from build123d import *

# Parameters (mm, degrees)
F0_R     = 5
F1_DEPTH = 3
F2_R     = 15
F3_DEPTH = 3
F4_R     = 17.221585
F5_DEPTH = 25


with BuildPart() as f1:
    # F0 (on Front) → F1 (new body)
    with BuildSketch(Plane.XZ):
        Circle(F0_R)
    extrude(amount=F1_DEPTH)

    # F2 (on face) → F3 (join)
    with BuildSketch(Plane.XZ.offset(3)):
        Circle(F2_R)
    extrude(amount=F3_DEPTH)

    # F4 (on face) → F5 (cut)
    with BuildSketch(Plane.XZ.offset(6)):
        Circle(F4_R)
        Polygon((-9.586422, 12.19146), (-0.589618, 15.497856), (8.6324, 12.884598), (14.557135, 5.349861), (14.921539, -4.228341), (9.586422, -12.19146), (0.589618, -15.497856), (-8.6324, -12.884598), (-14.557135, -5.349861), (-14.921539, 4.228341), align=None, mode=Mode.SUBTRACT)
    extrude(amount=-F5_DEPTH, mode=Mode.SUBTRACT)


solid = f1.part
Here's how the part is built. I have some questions about the finished solid (model axes, mm). Give positions to 0.01 mm unless a question says otherwise; leave off trailing zeros. Loops run counter-clockwise (first coordinate to the right, second up) from the corner with the lowest first, then second, coordinate; pieces in that order, holes last. Notation, with made-up numbers: (78.5, 4.25) -> (112.5, 4.25) arc R8 ccw to (112.5, 14.25) -> close; hole circle Ø9 at (83, -29.75). An arc over 180 degrees is marked (long way). Answer as a JSON object with one key per item and string values. Group by question number.
Item 1: I need wall thicknesses on L1, parallel to Y at x = 6.25, z = 3.75; L2, parallel to X at y = -4.85, z = 2.25; L3, parallel to X at y = -5.8, z = -12.5. Which ranges of each line are inside material? Lowest first, please.
Item 2: Will these pins go through, and if not, where does the flat tip stop? pin 1 (5 mm diameter, centred on x = -3.5, z = -11, fed in from +Y); pin 2 (3 mm diameter, centred on x = 6, y = -2.5, fed in from +Z).
Item 3: Imagine slicing it at B-B on x = 0. Write out the boundary of the cut face in (y, z).
Item 4: Imagine slicing it at C-C on z = 0. Write out the boundary of the cut face in (x, y), then the cut area to 3 significant figures.
Item 5: Imagine slicing it at A-A on y = -3.6. Write out the boundary of the cut face in (x, z).
Item 6: Imagine slicing it at D-D on y = -1.2. Write out the boundary of the cut face in (x, z), then the cut area to 3 significant figures.
Answer list:
{
 "1": {"L1": "y = -6 to -3", "L2": "x = -14.83 to 14.68", "L3": "x = -8.29 to 8.29"},
 "2": {"pin 1": "stops at y = -3", "pin 2": "stops at z = 14.03"},
 "3": {"outline": "(-6, -15) -> (-3, -15) -> (-3, -5) -> (0, -5) -> (0, 5) -> (-3, 5) -> (-3, 15) -> (-6, 15) -> close"},
 "4": {"outline": "(-14.76, -6) -> (14.76, -6) -> (14.76, -3) -> (5, -3) -> (5, 0) -> (-5, 0) -> (-5, -3) -> (-14.76, -3) -> close", "area": "119 mm2"},
 "5": {"outline": "(-14.84, 2.16) -> (-14.64, -3.29) arc R15 ccw to (-13.28, -6.97) -> (-9.91, -11.26) arc R15 ccw to (-6.65, -13.45) -> (-1.4, -14.93) arc R15 ccw to (2.53, -14.79) -> (7.65, -12.9) arc R15 ccw to (10.74, -10.48) -> (13.77, -5.94) arc R15 ccw to (14.84, -2.16) -> (14.64, 3.29) arc R15 ccw to (13.28, 6.97) -> (9.91, 11.26) arc R15 ccw to (6.65, 13.45) -> (1.4, 14.93) arc R15 ccw to (-2.53, 14.79) -> (-7.65, 12.9) arc R15 ccw to (-10.74, 10.48) -> (-13.77, 5.94) arc R15 ccw to start"},
 "6": {"outline": "circle Ø10 at (0, 0)", "area": "78.5 mm2"}
}
